Can you work these out from the model? Positions are in its coordinate system, mm. Give positions to 0.01 mm unless a question says otherwise; leave off trailing zeros. Order: outer loops, then holes, each group sorted by start corner. A loop starts at its lowest first (then second) coordinate and runs counter-clockwise, first axis right, second up. Notation, with made-up numbers: M -27.75,66.5 L -6.75,66.5 A15 cw -6.75,77.5 Z; hole C -20.75,33 d8. An arc over 180 degrees is marked long. Write each question's results on one line, items separated by ' | '.
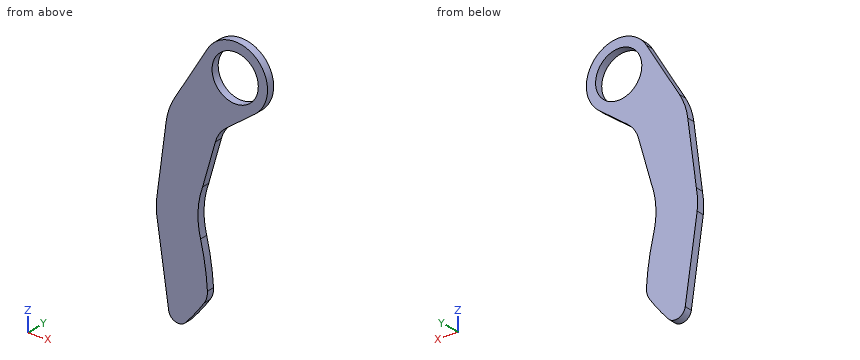
from build123d import *

# Parameters (mm, degrees)
SKETCH1_R           = 15
BOSS_EXTRUDE2_DEPTH = 5


with BuildPart() as part:
    # Sketch1 → Boss-Extrude2 (new body)
    with BuildSketch(Plane(origin=(0, 0, 0), x_dir=(1, 0, 0), z_dir=(0, 1, 0))):
        with BuildLine():
            Line((12.766893669, 16.673524704), (-5.806288098, 30.894983029))
            ThreePointArc((-5.806288098, 30.894983029), (-10.173884932, 35.51072238), (-12.873087905, 41.263569952))
            Line((-12.873087905, 41.263569952), (-21.139528525, 70.102189189))
            ThreePointArc((-21.139528525, 70.102189189), (-24.1253581, 85.250444887), (-22.456551163, 100.599709115))
            ThreePointArc((-22.456551163, 100.599709115), (-19.558480324, 114.843106453), (-18.020623668, 129.29676271))
            ThreePointArc((-18.020623668, 129.29676271), (-18.441772746, 133.226047543), (-20.116399197, 136.805470974))
            ThreePointArc((-20.116399197, 136.805470974), (-25.866377757, 144.615905974), (-32.098124488, 152.047627243))
            ThreePointArc((-32.098124488, 152.047627243), (-38.706331156, 153.910886754), (-43.194615771, 148.715173848))
            Line((-43.194615771, 148.715173848), (-50.932711484, 96.056215067))
            ThreePointArc((-50.932711484, 96.056215067), (-51.118515181, 89.191813761), (-50.383474997, 82.364351257))
            Line((-50.383474997, 82.364351257), (-44.824882263, 40.292034954))
            ThreePointArc((-44.824882263, 40.292034954), (-42.933064202, 32.343713579), (-39.465684055, 24.945601445))
            Line((-39.465684055, 24.945601445), (-18.005501401, -10.807493664))
            ThreePointArc((-18.005501401, -10.807493664), (13.987935708, -15.66325811), (12.766893669, 16.673524704))
        make_face()
        with Locations(Location((0, 0, 0), (0, 0, 270))):
            Circle(SKETCH1_R, mode=Mode.SUBTRACT)
    extrude(amount=BOSS_EXTRUDE2_DEPTH)


solid = part.part
(1) Imagine slicing it at B-B, the plane y = 4.2. Write out the boundary of the cut face in (x, z), plus the area to 3 significant figures.
Data:
outline: M -50.93,-96.06 L -43.19,-148.72 A6.4 ccw -32.1,-152.05 A153.5 ccw -20.12,-136.81 A12 ccw -18.02,-129.3 A153.5 ccw -22.46,-100.6 A51.17 cw -21.14,-70.1 L -12.87,-41.26 A20 cw -5.81,-30.89 L 12.77,-16.67 A21 ccw long -18.01,10.81 L -39.47,-24.95 A40 ccw -44.82,-40.29 L -50.38,-82.36 A51.17 ccw Z; hole C 0,0 d30 | area: 4,740 mm2
(2) Will these pins go through, and if not, where does the flat tip stop? P1, Ø1, axis at x = -17.5, y = 3.5, coming from the +Z side; P2, Ø24, axis at x = 0, z = 0, coming from the -Y side; P3, Ø1, axis at y = 1, z = -7.5, coming from the -X side.
Data:
P1: stops at z = 12.33 | P2: passes through | P3: stops at x = -29.29
(3) I need wall thicknesses on L1, parallel to X at y = 1.05, z = 0; L2, parallel to X at y = 0.7, z = 1; L3, parallel to X at y = 1.7, z = -107. Which ranges of each line are inside material? Lowest first, please. Write a range as from..to.
Data:
L1: x = -24.49..-15, 15..21 | L2: x = -23.89..-14.97, 14.97..20.98 | L3: x = -49.32..-20.98
(4) Imagine slicing it at D-D, the plane x = -27.5. Write out the boundary of the cut face in (y, z), plus the area to 3 significant figures.
Data:
outline: M 0,-146.66 L 5,-146.66 L 5,-5.01 L 0,-5.01 Z | area: 708 mm2
(5) Imagine slicing it at A-A, the plane x = 3.5. Write out the boundary of the cut face in (y, z).
Data:
outline: M 0,-23.77 L 5,-23.77 L 5,-14.59 L 0,-14.59 Z; M 0,14.59 L 5,14.59 L 5,20.71 L 0,20.71 Z
(6) Imagine slicing it at C-C, the plane z = 0. Write out the boundary of the cut face in (x, y), plus the area to 3 significant figures.
Data:
outline: M -24.49,0 L -15,0 L -15,5 L -24.49,5 Z; M 15,0 L 21,0 L 21,5 L 15,5 Z | area: 77.5 mm2
